```python
from build123d import *

# Parameters (mm, degrees)
SKETCH1_R           = 25
BOSS_EXTRUDE1_DEPTH = 2
SKETCH2_R           = 5
BOSS_EXTRUDE2_DEPTH = 4
SKETCH3_R           = 2.1
CUT_EXTRUDE1_DEPTH  = 20
SKETCH4_R           = 4.5
CUT_EXTRUDE2_DEPTH  = 5
SKETCH5_R           = 2.25
CUT_EXTRUDE3_DEPTH  = 10
BOSS_EXTRUDE3_START = 1.5
SKETCH6_R           = 25
SKETCH6_R_2         = 4.5
BOSS_EXTRUDE3_DEPTH = 1.5
BOSS_EXTRUDE5_START = 3.5
SKETCH7_R           = 4.5
SKETCH7_R_2         = 2.25
BOSS_EXTRUDE5_DEPTH = 3.5


with BuildPart() as part:
    # Sketch1 → Boss-Extrude1 (new body)
    with BuildSketch(Plane(origin=(0, 0, 0), x_dir=(1, 0, 0), z_dir=(0, 1, 0))):
        with Locations(Location((0, 0, 0), (0, 0, 270))):
            Circle(SKETCH1_R)
    extrude(amount=BOSS_EXTRUDE1_DEPTH)

    # Sketch2 → Boss-Extrude2 (add)
    with BuildSketch(Plane(origin=(0, 2, 0), x_dir=(1, 0, 0), z_dir=(0, 1, 0))):
        with Locations(Location((0, 0, 0), (0, 0, 270))):
            Circle(SKETCH2_R)
    extrude(amount=BOSS_EXTRUDE2_DEPTH)

    # Sketch3 → Cut-Extrude1 (cut)
    with BuildSketch(Plane.XZ):
        with Locations(Location((0, 0, 0), (0, 0, 270))):
            Circle(SKETCH3_R)
    extrude(amount=-CUT_EXTRUDE1_DEPTH, mode=Mode.SUBTRACT)

    # Sketch4 → Cut-Extrude2 (cut)
    with BuildSketch(Plane.XZ):
        with Locations(Location((0, 0, 0), (0, 0, 270))):
            Circle(SKETCH4_R)
    extrude(amount=-CUT_EXTRUDE2_DEPTH, mode=Mode.SUBTRACT)

    # Sketch5 → Cut-Extrude3 (cut)
    with BuildSketch(Plane.XZ.offset(-5)):
        with Locations(Location((0, 0, 0), (0, 0, 270))):
            Circle(SKETCH5_R)
    extrude(amount=-CUT_EXTRUDE3_DEPTH, mode=Mode.SUBTRACT)

    # Sketch6 → Boss-Extrude3 (add)
    with BuildSketch(Plane.XZ.offset(BOSS_EXTRUDE3_START)):
        with Locations(Location((0, 0, 0), (0, 0, 270))):
            Circle(SKETCH6_R)
        with Locations(Location((0, 0, 0), (0, 0, 270))):
            Circle(SKETCH6_R_2, mode=Mode.SUBTRACT)
    extrude(amount=-BOSS_EXTRUDE3_DEPTH)

    # Sketch7 → Boss-Extrude5 (add)
    with BuildSketch(Plane.XZ.offset(-5).offset(BOSS_EXTRUDE5_START)):
        with Locations(Location((0, 0, 0), (0, 0, 270))):
            Circle(SKETCH7_R)
        with Locations(Location((0, 0, 0), (0, 0, 270))):
            Circle(SKETCH7_R_2, mode=Mode.SUBTRACT)
    extrude(amount=-BOSS_EXTRUDE5_DEPTH)


solid = part.part
```
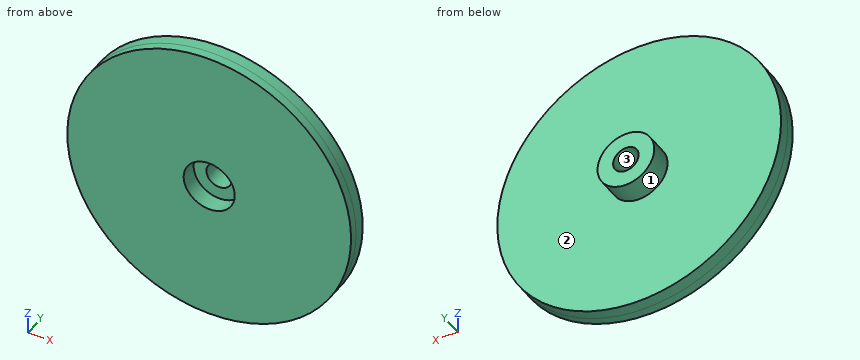
Geometry check sheet. Reference: the model listing, model coordinates, mm. Face numbers are marked on the shaded views. Coordinates: 2 decimals unless noted, no trailing zeros. Write each loop counter-clockwise with the first axis right and the second up, starting at its lowest first coordinate (ties: lowest second). Pieces come first, ordered by that corner, then holes. Notation, with made-up numbers: (-15, 75) -> (23, 75) arc R25 cw to (23, 93) -> close; hole circle Ø6 at (-39, -30.5). An arc over 180 degrees is marked (long way). Use CSV: the item, a comma, the result in double quotes. Start each with the question number.
Item 1: Mould release check, pull along Z, two halves, no side actions. Record for the marked faces 1, 2 and 3: released by +Z, released by -Z, zero draft, split by the parting line, or undercut.
Item 2: Cross-section at C-C, the plane y = 3. Record the cut outline in (x, z).
Item 3: Cross-section at D-D, the plane z = -16. Record the cut outline in (x, y), plus the area to 3 significant figures.
Item 4: Cross-section at B-B, the plane z = 0. Record the cut outline in (x, y).
Item 5: Thickness scan on line 1 (X direction, y = 0.7, z = 0); line 2 (X direction, y = 3.1, z = 0); line 3 (Y direction, x = 3, z = -18.5). Record the ranges inside material, lowest first.
Item 6: Cross-section at A-A, the plane x = 0. Record the cut outline in (y, z).
Item 7: Depth check by flat-ended pin: pin 1 Ø7 at (x, z) = (-0.5, 1.5) entering from -Y; pin 2 Ø2.5 at (x, z) = (0, 0) entering from +Y; pin 3 Ø10 at (x, z) = (12.5, 10) entering from +Y. Enter the tip coordinate at first touch or a pass-through.
Answers:
1,face 1,"split by the parting line"
1,face 2,"zero draft"
1,face 3,"undercut"
2,outline,"circle Ø10 at (0, 0); hole circle Ø4.5 at (0, 0)"
3,outline,"(-19.21, -1.5) -> (19.21, -1.5) -> (19.21, 2) -> (-19.21, 2) -> close"
3,area,"134 mm^2"
4,outline,"(-25, -1.5) -> (-4.5, -1.5) -> (-4.5, 1.5) -> (-2.25, 1.5) -> (-2.25, 6) -> (-5, 6) -> (-5, 2) -> (-25, 2) -> close; (2.25, 1.5) -> (4.5, 1.5) -> (4.5, -1.5) -> (25, -1.5) -> (25, 2) -> (5, 2) -> (5, 6) -> (2.25, 6) -> close"
5,line 1,"-25 to -4.5, 4.5 to 25"
5,line 2,"-5 to -2.25, 2.25 to 5"
5,line 3,"-1.5 to 2"
6,outline,"(-1.5, -25) -> (2, -25) -> (2, -5) -> (6, -5) -> (6, -2.25) -> (1.5, -2.25) -> (1.5, -4.5) -> (-1.5, -4.5) -> close; (-1.5, 4.5) -> (1.5, 4.5) -> (1.5, 2.25) -> (6, 2.25) -> (6, 5) -> (2, 5) -> (2, 25) -> (-1.5, 25) -> close"
7,pin 1,"y = -1.5"
7,pin 2,"through"
7,pin 3,"y = 2"
